Check sheet for the modelled part. Datum: model origin and axes. Units: mm. A direction names the side the tool comes from. Round coordinates to 2 decimals unless told otherwise and drop trailing zeros. Loops run counter-clockwise (first coordinate to the right, second up) from the corner with the lowest first, then second, coordinate; pieces in that order, holes last. Notation, with made-up numbers: (0, 3) - (52, 3) arc R30 cw to (52, 27) - close; hole circle Ø6 at (50, 64). An arc over 180 degrees is marked (long way). Return JSON: item names as keys, results as strings.
from build123d import *

# Parameters (mm, degrees)
SKETCH_1_R          = 14
EXTRUDE_1_DEPTH     = 13
SKETCH_2_R          = 22.5
EXTRUDE_2_DEPTH     = 7
EXTRUDE_3_DEPTH     = 13
SKETCH_4_R          = 14
CUT_EXTRUDE_1_DEPTH = 40
CUT_EXTRUDE_2_DEPTH = 41


with BuildPart() as part:
    # 草图1 → 凸台-拉伸1 (new body)
    with BuildSketch(Plane.XY):
        with BuildLine():
            ThreePointArc((0, 22.5), (-22.5, 0), (0, -22.5))
            add(Edge.make_bspline(
                [(0, 22.5), (3.74256312, 22.5), (25.152008405, 16.944120599), (65.295682957, 0), (25.155025761, -16.944120599), (3.738346709, -22.5), (0, -22.5)],
                knots=[0, 0, 0, 0, 0.192196215, 0.5, 0.807803785, 1, 1, 1, 1], degree=3))
        make_face()
        Circle(SKETCH_1_R, mode=Mode.SUBTRACT)
    extrude(amount=EXTRUDE_1_DEPTH)

    # 草图2 → 凸台-拉伸2 (add)
    with BuildSketch(Plane.XY.offset(13)):
        Circle(SKETCH_2_R)
    extrude(amount=EXTRUDE_2_DEPTH)

    # 草图3 → 凸台-拉伸3 (add)
    with BuildSketch(Plane.XY.offset(20)):
        with BuildLine():
            ThreePointArc((22.5, 0), (0, 22.5), (-22.5, 0))
            add(Edge.make_bspline(
                [(22.5, 0), (22.5, -3.74256312), (16.944120599, -25.152008405), (0, -65.295682957), (-16.944120599, -25.155025761), (-22.5, -3.738346709), (-22.5, 0)],
                knots=[0, 0, 0, 0, 0.192196215, 0.5, 0.807803785, 1, 1, 1, 1], degree=3))
        make_face()
    extrude(amount=EXTRUDE_3_DEPTH)

    # 草图4 → 切除-拉伸1 (cut)
    with BuildSketch(Plane(origin=(0, 0, 13), x_dir=(-1, 0, 0), z_dir=(0, 0, -1))):
        Circle(SKETCH_4_R)
    extrude(amount=-CUT_EXTRUDE_1_DEPTH, mode=Mode.SUBTRACT)

    # 草图5 → 切除-拉伸2 (cut)
    with BuildSketch(Plane.XY.offset(33)):
        Polygon((-4, -14), (-4, -9.153591973), (4, -9.153591973), (4, -14), (4, -17.2), (-4, -17.2), align=None)
    extrude(amount=-CUT_EXTRUDE_2_DEPTH, mode=Mode.SUBTRACT)


solid = part.part
Q1. Depth check by flat-ended pin: P1, Ø5, axis at y = -3, z = 10, coming from the +X side; P2, Ø4, axis at y = -14.5, z = 19, coming from the +X side; P3, Ø12, axis at x = 25.5, z = 12, coming from the -Y side. Enter the tip coordinate at first touch or a pass-through.
Answer key:
{"P1": "stops at x = 49.97", "P2": "stops at x = 19.93", "P3": "stops at y = -17.89"}
Q2. Scan lines: probe 1 along Y at (x, z) = (0, 12); probe 2 along X at (y, z) = (0, 8); probe 3 along Z at (x, y) = (14.5, -18). Record each from-to range of solid material in increasing order. Write a range as [from, to].
Answer key:
{"probe 1": "y = [-22.5, -17.2], [14, 22.5]", "probe 2": "x = [-22.5, -14], [14, 50]", "probe 3": "z = [0, 13], [20, 33]"}
Q3. Sectioned sample at A-A (z = 16). Enter the section's corners in (x, y), plus the area to 3 significant figures.
Answer key:
{"outline": "circle Ø45 at (0, 0); hole (-4, -17.2) - (4, -17.2) - (4, -13.42) arc R14 ccw (long way) to (-4, -13.42) - close", "area": "948 mm²"}
Q4. Draft check along Y on faces 1 (the face through (0, -31, 20)), 2 (the face through (-16.58, 15.21, 16.27)), 3 (the face through (0, -17.2, 17)). Enter one of: released by +Y, released by -Y, zero draft, split by the parting line, or undercut.
Answer key:
{"face 1": "zero draft", "face 2": "split by the parting line", "face 3": "undercut"}
Q5. Tool access check on faces 4 (the face through (4, -15, 17)), 5 (the face through (11, 10, 0)). Record the directions out of +Z, -Z, +X, -X, +Y, -Y that give a thin tool (end or side, any length) a straight path to the whole face; none if there is none.
Answer key:
{"face 4": "+Z, -Z", "face 5": "-Z, +X, -X, +Y, -Y"}
